Autodesk Inventor part; units mm, degrees
ref_plane "YZ Plane" through (0, 0, 0) normal (1, 0, 0) x (0, 1, 0)
ref_plane "XZ Plane" through (0, 0, 0) normal (0, 1, 0) x (-1, 0, 0)
ref_plane "XY Plane" through (0, 0, 0) normal (0, 0, 1) x (1, 0, 0)
sketch "Sketch1" plane through (0, 0, 0) normal (0, 1, 0) x (-1, 0, 0)
  line L0 (0, 0) -> (43.2562, 0)
  line L1 (43.2562, 0) -> (43.2562, -54.991)
  line L2 (43.2562, -54.991) -> (0, -54.991)
  line L3 (0, -54.991) -> (0, 0)
  dimension "d0" = 43.2562
  dimension "d1" = 54.991
extrude "Extrusion1" add sketch "Sketch1" along normal blind 0.5
sketch "Sketch2" plane through (0, 0.5, 0) normal (0, 1, 0) x (1, 0, 0)
  circle A0 centre (-42.4688, 0.7874) radius 0.381
  circle A1 centre (-42.4688, 54.2036) radius 0.381
  circle A2 centre (-0.7874, 54.2036) radius 0.381
  circle A3 centre (-0.7874, 0.7874) radius 0.381
  point P0 (0, 0)
  dimension "d4" = 0.762
  dimension "d5" = 0.762
  dimension "d6" = 0.762
  dimension "d10" = 0.762
extrude "Extrusion2" add sketch "Sketch2" along normal blind 1.905 contours A0 | A1 | A2
fillet "Fillet1" radius 0.2286 10 edges at (-42.8498, 2.405, -0.7874) (-42.8498, 2.405, -54.2036) (-1.1684, 2.405, -54.2036) (-1.1684, 0.5, -54.2036) (-42.8498, 0.5, -54.2036) (-42.8498, 0.5, -0.7874) (-21.6281, 0, 0) (0, 0, -27.4955) (-21.6281, 0, -54.991) (-43.2562, 0, -27.4955)
sketch "Sketch3" plane through (0, 0.5, 0) normal (0, 1, 0) x (1, 0, 0)
  line L0 (0, 54.991) -> (-43.2562, 54.991)
  line L1 (0, 54.991) -> (0, 25.019)
  line L2 (0, 54.991) -> (0, 0)
  line L3 (0, 25.019) -> (-2.8956, 25.019)
  line L4 (-43.2562, 25.019) -> (-40.3606, 25.019)
  line L5 (-40.3606, 25.019) -> (-39.3606, 25.019)
  point P0 (-38.9037, 23.6963)
  dimension "d11" = 29.972
  dimension "d12" = 2.8956
  dimension "d20" = 2.8956
  dimension "d21" = 1
hole "Hole1" at (-38.9037, 0.5, -23.6963) direction (0, -1, 0) diameter 2 end through all
properties part number "enclosure_lid"
Verification items for the finished model (mm, model axes). Give positions to 0.01 mm unless a question says otherwise; leave off trailing zeros. Order: outer loops, then holes, each group sorted by start corner. A loop starts at its lowest first (then second) coordinate and runs counter-clockwise, first axis right, second up. Notation, with made-up numbers: M 5,-36.75 L 30,-36.75 A10 ccw 30,-18.75 Z; hole C 63.5,-20 d11. An arc over 180 degrees is marked long. Return JSON: item names as keys, results as strings. Group by question number.
1) Go/stop test with flat-tipped pins: pin 1 Ø4 at (x, z) = (-37, -18.5) entering from +Y; pin 2 Ø1.5 at (x, z) = (-31.5, -13) entering from -Y. Record where each tip stops, or that it passes through.
2) Section check A-A on x = -34.5. Record the cut outline in (y, z), and give its area (3 significant figures).
3) Scan lines: line 1 (Y direction, x = -28, z = -39.5); line 2 (Z direction, x = -16, y = 0.2); line 3 (Z direction, x = -38.5, y = 0.35). Record each from-to range of solid material in increasing order.
4) Section check B-B on z = -43. Record the cut outline in (x, y), and give its area (3 significant figures).
5) Mould release check, pull along Z, two halves, no side actions. Record for faces 1 (the face through (-21, 0, -27)), 2 (the face through (-37.927, 0.246, -23.913)): pulls with the +Z half, pulls with the -Z half, needs draft (parallel to the pull), parting line crosses it, or undercut.
Answer block:
{
 "1": {"pin 1": "stops at y = 0.5", "pin 2": "stops at y = 0"},
 "2": {"outline": "M 0,-54.76 A0.23 ccw 0.23,-54.99 L 0.5,-54.99 L 0.5,0 L 0.23,0 A0.23 ccw 0,-0.23 Z", "area": "27.5 mm^2"},
 "3": {"line 1": "y = 0 to 0.5", "line 2": "z = -54.99 to 0", "line 3": "z = -54.99 to -24.61, -22.78 to 0"},
 "4": {"outline": "M -43.26,0.23 A0.23 ccw -43.03,0 L -0.23,0 A0.23 ccw 0,0.23 L 0,0.5 L -43.26,0.5 Z", "area": "21.6 mm^2"},
 "5": {"face 1": "needs draft", "face 2": "undercut"}
}
